Can you work these out from the model? Positions are in its coordinate system, mm. Round coordinates to 2 decimals unless told otherwise and drop trailing zeros. Loops run counter-clockwise (first coordinate to the right, second up) from the corner with the lowest first, then second, coordinate; pieces in that order, holes last. Notation, with made-up numbers: (-20, 42.25) -> (-12, 42.25) arc R20 ccw to (-12, 64.25) -> close; hole circle Ø2 at (18.25, 80.5). An arc over 180 degrees is marked (long way). Write item = value, one per line.
from build123d import *

# Parameters (mm, degrees)
F0_R     = 1.1
F1_DEPTH = 1.5
F2_R     = 1.1
F3_DEPTH = 1.5
F4_R     = 1
F5_SIZE  = 5
F6_R     = 1


with BuildPart() as f1:
    # F0 (on Top) → F1 (new body)
    with BuildSketch(Plane.XY):
        with BuildLine():
            Line((7.5, -55), (7.5, 55))
            Line((7.5, 55), (-7.5, 55))
            Line((-7.5, 55), (-7.5, 50.25))
            Line((-7.5, 50.25), (-4.5, 50.25))
            ThreePointArc((-4.5, 50.25), (0.75, 45), (-4.5, 39.75))
            Line((-4.5, 39.75), (-7.5, 39.75))
            Line((-7.5, 39.75), (-7.5, 28))
            Line((-7.5, 28), (-42.5, 28))
            Line((-42.5, 28), (-42.5, -55))
            Line((-42.5, -55), (-7.5, -55))
            Line((-7.5, -55), (7.5, -55))
        make_face()
        with Locations((-4.5, 38)):
            Circle(F0_R, mode=Mode.SUBTRACT)
        with Locations((0.4497474683, 40.0502525317)):
            Circle(F0_R, mode=Mode.SUBTRACT)
        with Locations((-4.5, 52)):
            Circle(F0_R, mode=Mode.SUBTRACT)
        with Locations((0.4497474683, 49.9497474683)):
            Circle(F0_R, mode=Mode.SUBTRACT)
        with Locations((2.5, 45)):
            Circle(F0_R, mode=Mode.SUBTRACT)
    extrude(amount=F1_DEPTH)

    # F2 (on face) → F3 (cut, through all)
    with BuildSketch(Plane.XY.offset(1.5)):
        Polygon((7.5, -55), (7.5, 23), (-5.5, 3), (-17.5, 3), (-17.5, 28), (-42.5, 28), (-42.5, -55), align=None)
        with Locations((-12.5, 23)):
            Circle(F2_R)
        with Locations((-12.5, 8)):
            Circle(F2_R)
    extrude(amount=-F3_DEPTH, mode=Mode.SUBTRACT)

    # F4
    f4_edges = [f1.edges().sort_by_distance(p)[0] for p in [
        (-17.5, 3, 0.75),
        (-5.5, 3, 0.75),
        (7.5, 23, 0.75),
        (-7.5, 50.25, 0.75),
        (-7.5, 55, 0.75),
        (-7.5, 39.75, 0.75),
        (-17.5, 28, 0.75),
    ]]
    fillet(f4_edges, radius=F4_R)

    # F5
    f5_edges = [f1.edges().sort_by_distance(p)[0] for p in [
        (7.5, 55, 0.75),
        (-7.5, 28, 0.75),
    ]]
    chamfer(f5_edges, length=F5_SIZE)

    # F6
    f6_edges = [f1.edges().sort_by_distance(p)[0] for p in [
        (-7.5, 33, 0.75),
        (-12.5, 28, 0.75),
        (2.5, 55, 0.75),
        (7.5, 50, 0.75),
    ]]
    fillet(f6_edges, radius=F6_R)


solid = f1.part
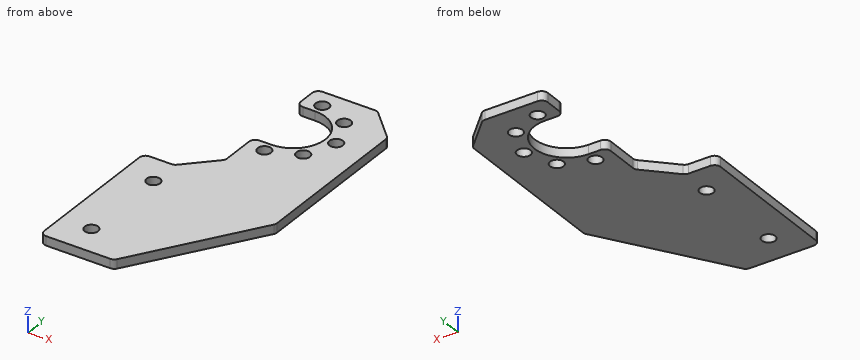
1. Suppose I cut it at D-D, the plane x = -10.5. List the corners of the cut face in (y, z) for me.
Entries:
outline = (3, 0) -> (30, 0) -> (30, 1.5) -> (3, 1.5) -> close
2. Suppose I cut it at A-A, the plane y = 8. List the corners of the cut face in (x, z) for me, and give its area (3 significant figures).
Entries:
outline = (-17.5, 0) -> (-13.6, 0) -> (-13.6, 1.5) -> (-17.5, 1.5) -> close; (-11.4, 0) -> (-2.25, 0) -> (-2.25, 1.5) -> (-11.4, 1.5) -> close
area = 19.6 mm²
3. I'm going to push a flat-ended pin straight in: pin 1 (1.3 mm diameter, centred on x = -12.5, y = 8, fed in from +Z). Where does the tip first touch, or does it pass through?
Entries:
pin_1 = through
4. Suppose I cut it at C-C, the plane y = 52. List the corners of the cut face in (x, z) for me, and give its area (3 significant figures).
Entries:
outline = (-7.5, 0) -> (-5.6, 0) -> (-5.6, 1.5) -> (-7.5, 1.5) -> close; (-3.4, 0) -> (5.5, 0) -> (5.5, 1.5) -> (-3.4, 1.5) -> close
area = 16.2 mm²
5. Suppose I cut it at B-B, the plane z = 0.8. Count the separate pieces of the cut face and the enclosed holes in it, and give its area (3 significant figures).
Entries:
separate_pieces = 1
enclosed_holes = 7
area = 797 mm²
6. I need wall thicknesses on line 1 (Y direction, x = 0, z = 0.6); line 2 (Y direction, x = -13.5, z = 0.4); line 3 (Y direction, x = -5.25, z = 0.65). Which ranges of each line are inside material? Lowest first, please. Write a range as [from, to].
Entries:
line_1 = [11.46, 39.05], [41.05, 42.3], [47.7, 48.95], [50.95, 55]
line_2 = [3, 7.54], [8.46, 22.54], [23.46, 28]
line_3 = [3.39, 37.2], [38.8, 39.75], [50.25, 51.2], [52.8, 55]
